Geometry check sheet. Reference: the model listing, model coordinates, mm. A direction names the side the tool comes from. Give positions to 0.01 mm unless a question says otherwise; leave off trailing zeros. Write each loop counter-clockwise with the first axis right and the second up, starting at its lowest first coordinate (ties: lowest second). Pieces come first, ordered by that corner, then holes. Notation, with made-up numbers: M 20,-34.75 L 50,-34.75 A22 cw 50,-9.75 Z; hole C 87,-11.75 d9. An arc over 180 degrees is marked long. One line per item, written item: value. Start each with the question number.
1. Cross-section at B-B on y = 0.25. Record the cut outline in (x, z) (3 decimals), then the cut area to 3 significant figures.
2. Tool access check on faces 4 (the face through (1.293, -1.246, -16.043)), 5 (the face through (-1.29, -1.25, -14.03)), 6 (the face through (0.1, 1.2, -17.4)), 7 (the face through (-1, -1, -16)). Record the directions out of +Z, -Z, +X, -X, +Y, -Y that give a thin tool (end or side, any length) a straight path to the whole face; none if there is none.
3. Cross-section at A-A on x = 0. Record the cut outline in (y, z) (3 decimals), then the cut area to 3 significant figures.
4. Gauge pin test, flat ends, axial feed: pin 1 (4.5 mm diameter, centred on x = 0, z = 0, fed in from +Y); pin 2 (6 mm diameter, centred on x = 4, z = -7, fed in from -Y); pin 3 (1.5 mm diameter, centred on x = 4.5, y = -0.5, fed in from +Z). Record the tip position at first contact, or that the pin passes through.
5. Scan lines: line 1 (X direction, y = 0.5, z = 0) (3 decimals); line 2 (Y direction, x = 2.75, z = -6.25); line 3 (X direction, y = 0.05, z = 0.75). Record each from-to range of solid material in increasing order.
6. Cross-section at C-C on z = -12.5. Record the cut outline in (x, y), then the cut area to 3 significant figures.
7. Cross-section at D-D on x = 3.5. Record the cut outline in (y, z), then the cut area to 3 significant figures.
8. Release check for a two-part mould opening along Y. For faces 1 (the face through (0, 1, 6)), 2 (the face through (0, -1.5, -15)), 3 (the face through (-0.05, -0.49, -16.08)) record: pulls with the +Y half, pulls with the -Y half, needs draft (parallel to the pull), parting line crosses it, or undercut.
from build123d import *

# Parameters (mm, degrees)
SKETCH1_R           = 2.525
BOSS_EXTRUDE1_DEPTH = 2.5
SKETCH2_R           = 1.040591752
BOSS_EXTRUDE2_DEPTH = 1
BOSS_EXTRUDE3_DEPTH = 0.5


with BuildPart() as part:
    # Sketch1 → Boss-Extrude1 (new body)
    with BuildSketch(Plane(origin=(0, 0, 0), x_dir=(1, 0, 0), z_dir=(0, 1, 0))):
        with BuildLine():
            Line((-5.520391153, 2.350591738), (-6, 0))
            ThreePointArc((-6, 0), (0, -6), (6, 0))
            Line((6, 0), (5.520391153, 2.350591738))
            Line((5.520391153, 2.350591738), (2.939437593, 15))
            ThreePointArc((2.939437593, 15), (0, 17.40024452), (-2.939437593, 15))
            Line((-2.939437593, 15), (-5.520391153, 2.350591738))
        make_face()
        with Locations(Location((0, 0, 0), (0, 0, 270))):
            Circle(SKETCH1_R, mode=Mode.SUBTRACT)
    extrude(amount=BOSS_EXTRUDE1_DEPTH)

    # Sketch2 → Boss-Extrude2 (add)
    with BuildSketch(Plane.XZ):
        with Locations(Location((0, -15.039011309, 0), (0, 0, 90))):
            Circle(SKETCH2_R)
    extrude(amount=BOSS_EXTRUDE2_DEPTH)

    # Sketch3 → Boss-Extrude3 (add)
    with BuildSketch(Plane.XZ.offset(1)):
        Polygon((1.147373963, -13.536920287), (-0.727162002, -13.294310799), (-1.874535964, -14.79640182), (-1.147373963, -16.54110233), (0.727162002, -16.783711818), (1.874535964, -15.281620797), align=None)
    extrude(amount=BOSS_EXTRUDE3_DEPTH)


solid = part.part
Report:
1. outline: M -6,0 L -2.939,-15 A3 ccw 2.939,-15 L 6,0 A6 ccw Z; hole C 0,0 d5.05
1. area: 181 mm^2
2. face 4: -Z, +X, -Y
2. face 5: +Z, -X, -Y
2. face 6: -Z, +Y, -Y
2. face 7: none
3. outline: M -1.5,-16.69 L -1,-16.69 L -1,-16.08 L 0,-16.08 L 0,-17.4 L 2.5,-17.4 L 2.5,-2.525 L 0,-2.525 L 0,-13.998 L -1,-13.998 L -1,-13.388 L -1.5,-13.388 Z; M 0,2.525 L 2.5,2.525 L 2.5,6 L 0,6 Z
3. area: 49.6 mm^2
4. pin 1: passes through
4. pin 2: stops at y = 0
4. pin 3: stops at z = 4.52
5. line 1: x = -6 to -2.525, 2.525 to 6
5. line 2: y = 0 to 2.5
5. line 3: x = -5.95 to -2.41, 2.41 to 5.95
6. outline: M -3.45,0 L 3.45,0 L 3.45,2.5 L -3.45,2.5 Z
6. area: 17.2 mm^2
7. outline: M 0,-12.25 L 2.5,-12.25 L 2.5,4.87 L 0,4.87 Z
7. area: 42.8 mm^2
8. face 1: needs draft
8. face 2: pulls with the -Y half
8. face 3: undercut
